Study the drawing (mm; zero at the part's minimum x, y, z) and answer. A direction names the side the tool comes from. Coordinates: 2 decimals unless noted, no trailing zeros. Loops run counter-clockwise (first coordinate to the right, second up) from the corner with the lowest first, then second, coordinate; pieces in that order, holes last. Notation, with made-up numbers: (25.5, 1) - (80.5, 1) arc R37 ccw to (80.5, 37) - close; hole circle Ø11 at (5.25, 23). An arc over 180 degrees is marked (long way). Use one line per item in the form item = value.
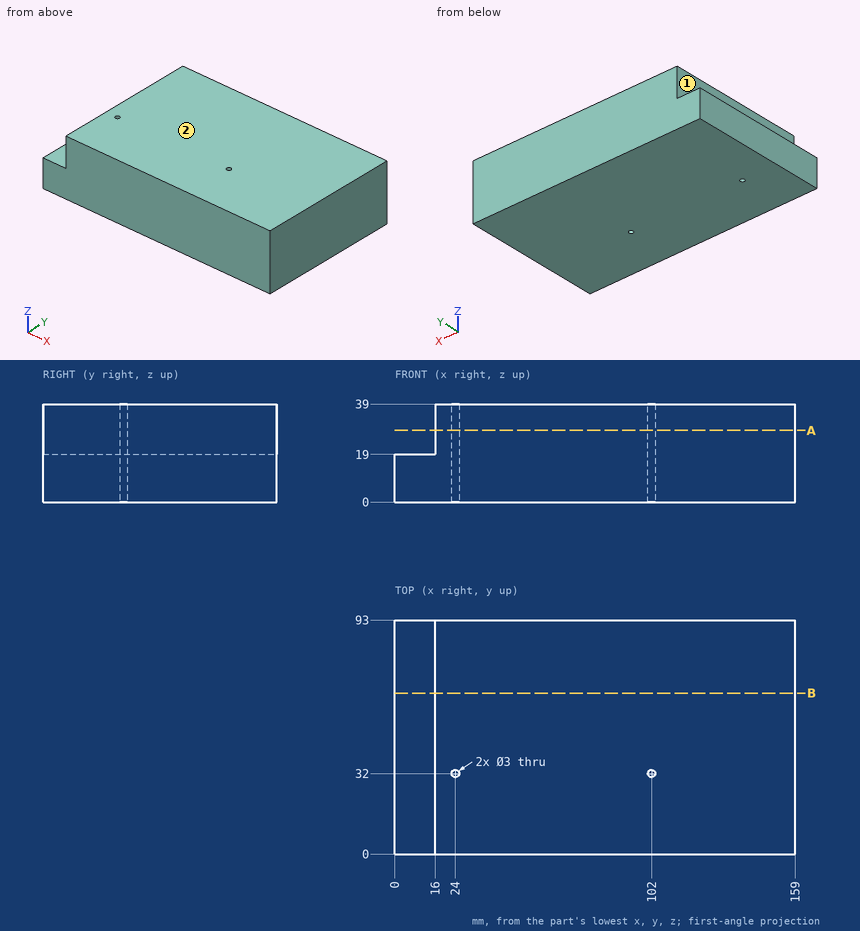
Item 1: Which of the six approach directions +Z, -Z, +X, -X, +Y, -Y give full straight-line access (tool end or side, diameter ignored) to the marked faces 1 and 2?
Results below:
face_1 = +Z, -X, +Y, -Y
face_2 = +Z, +X, -X, +Y, -Y
Item 2: The part is cut by section B-B on y = 64. Give the vertices of the cut face in (x, z).
Results below:
outline = (0, 0) - (159, 0) - (159, 39) - (16, 39) - (16, 19) - (0, 19) - close
Item 3: The part is cut by section A-A on z = 28.5. Give the vertices of the cut face in (x, y).
Results below:
outline = (16, 0) - (159, 0) - (159, 93) - (16, 93) - close; hole circle Ø3 at (24, 32); hole circle Ø3 at (102, 32)
Item 4: Find the intervals of material crossed by L1, parallel to Y at x = 24, z = 13; L2, parallel to X at y = 31, z = 22.5; L3, parallel to X at y = 26.5, z = 27.5, in increasing order.
Results below:
L1 = 0 to 30.5, 33.5 to 93
L2 = 16 to 22.88, 25.12 to 100.88, 103.12 to 159
L3 = 16 to 159
Item 5: Each of these flat-tipped pins is pushed along its axis until it touches: P1, Ø13, axis at x = 9, y = 51, coming from the +Z side; P2, Ø3, axis at x = 30, z = 29.5, coming from the -Y side; P3, Ø6, axis at y = 24.5, z = 31.5, coming from the -X side. Where does it stop, or does it pass through?
Results below:
P1 = 19
P2 = 0
P3 = 16
